```python
from build123d import *

# Parameters (mm, degrees)
F0_R     = 11.1
F0_R_2   = 10.983308
F1_DEPTH = 7
F2_R     = 45.72
F2_R_2   = 41.91
F3_DEPTH = 7


with BuildPart() as f1:
    # F0 (on Top) → F1 (new body)
    with BuildSketch(Plane.XY):
        with BuildLine():
            ThreePointArc((12.948403, 3.187646), (11.548449, 6.6675), (9.234784, 9.619823))
            Line((9.234784, 9.619823), (19.675505, 38.305468))
            ThreePointArc((19.675505, 38.305468), (0, 43.586091), (-19.675505, 38.305468))
            Line((-19.675505, 38.305468), (-9.234784, 9.619823))
            ThreePointArc((-9.234784, 9.619823), (-11.548449, 6.6675), (-12.948403, 3.187646))
            Line((-12.948403, 3.187646), (-43.011261, -2.113247))
            ThreePointArc((-43.011261, -2.113247), (-37.746662, -21.793046), (-23.335756, -36.192221))
            Line((-23.335756, -36.192221), (-3.713619, -12.807469))
            ThreePointArc((-3.713619, -12.807469), (0, -13.335), (3.713619, -12.807469))
            Line((3.713619, -12.807469), (23.335756, -36.192221))
            ThreePointArc((23.335756, -36.192221), (37.746662, -21.793046), (43.011261, -2.113247))
            Line((43.011261, -2.113247), (12.948403, 3.187646))
        make_face()
        with Locations((-22.404077, -12.935)):
            Circle(F0_R, mode=Mode.SUBTRACT)
        with BuildLine():
            ThreePointArc((8.382, 7.276818), (10.398322, 3.883928), (11.1, 0))
            ThreePointArc((11.1, 0), (-10.398322, -3.883928), (8.382, 7.276818))
        make_face(mode=Mode.SUBTRACT)
        with Locations((22.404077, -12.935)):
            Circle(F0_R_2, mode=Mode.SUBTRACT)
        with Locations((0, 25.87)):
            Circle(F0_R, mode=Mode.SUBTRACT)
    extrude(amount=F1_DEPTH)

    # F2 (on Top) → F3 (join)
    with BuildSketch(Plane.XY):
        Circle(F2_R)
        Circle(F2_R_2, mode=Mode.SUBTRACT)
    extrude(amount=F3_DEPTH)


solid = f1.part
```
Can you work these out from the model? Positions are in its coordinate system, mm. A direction names the side the tool comes from. Coordinates: 2 decimals unless noted, no trailing zeros. Write each loop counter-clockwise with the first axis right and the second up, starting at its lowest first coordinate (ties: lowest second). Pieces come first, ordered by that corner, then holes. Notation, with made-up numbers: M 8.25,31.25 L 14.25,31.25 A19 ccw 14.25,45.25 Z; hole C 6,69.25 d10. An arc over 180 degrees is marked long. Answer as CSV lines item,"result".
Item 1: I'm going to push flat-ended pins straight in: P1, Ø4, axis at x = -18.5, z = 2.5, coming from the -Y side; P2, Ø3, axis at x = 9, z = 2.5, coming from the +Y side; P3, Ø13.5, axis at x = 0, y = 0, coming from the +Z side; P4, Ø1.5, axis at x = 12, z = 5, coming from the +Y side. Where does each tip first touch, or does it pass through?
Geometry results:
P1,"stops at y = -42.64"
P2,"stops at y = 45.1"
P3,"passes through"
P4,"stops at y = 44.31"
Item 2: On a 3-axis mill with a long thin cutter (end or side, diameter ignored), from which of +Z, -Z, +X, -X, +Y, -Y can I reach the whole of each face in a straight line? I mean faces 4 (the flat face through (7, -10, 0)), 5 (the flat face through (13.02, -23.9, 3.45)). Say none if no direction works.
Geometry results:
face 4,"-Z, +X, -X, +Y, -Y"
face 5,"+Z, -Z"
Item 3: Imagine slicing it at B-B on y = 29. List the corners of the cut face in (x, z) for me, plus the area to 3 significant figures.
Geometry results:
outline,"M -35.35,0 L -30.26,0 L -30.26,7 L -35.35,7 Z; M -16.29,0 L -10.65,0 L -10.65,7 L -16.29,7 Z; M 10.65,0 L 16.29,0 L 16.29,7 L 10.65,7 Z; M 30.26,0 L 35.35,0 L 35.35,7 L 30.26,7 Z"
area,"150 mm2"
Item 4: We'd pull the mould along X, two halves only. Please class faces 1 (the flat face through (7, -10, 7)), 2 (the flat face through (-14.327, 23.61, 3.451)), 3 (the cylindrical face through (43.61, 13.73, 3.45)): +X half, -X half, draft (parallel to the pull), parting line (faces both ways), or undercut.
Geometry results:
face 1,"draft"
face 2,"undercut"
face 3,"parting line"
Item 5: Imagine slicing it at A-A on x = 0. List the corners of the cut face in (y, z) for me (3 decimals), plus the area to 3 significant figures.
Geometry results:
outline,"M -45.72,0 L -41.91,0 L -41.91,7 L -45.72,7 Z; M -13.335,0 L -11.1,0 L -11.1,7 L -13.335,7 Z; M 11.1,0 L 14.77,0 L 14.77,7 L 11.1,7 Z; M 36.97,0 L 45.72,0 L 45.72,7 L 36.97,7 Z"
area,"129 mm2"
Item 6: Imagine slicing it at D-D on z = 3. List the corners of the cut face in (x, y) for me (1 decimal), plus the area to 3 significant figures.
Geometry results:
outline,"C 0,0 d91.4; hole M -41.9,-1.9 L -12.9,3.2 A13.3 cw -9.2,9.6 L -19.3,37.2 A41.9 ccw Z; hole C -22.4,-12.9 d22.2; hole M -22.6,-35.3 A41.9 ccw 22.6,-35.3 L 3.7,-12.8 A13.3 cw -3.7,-12.8 Z; hole C 0,25.9 d22.2; hole M 8.4,7.3 A11.1 ccw long 11.1,0 A11.1 ccw Z; hole M 9.2,9.6 A13.3 cw 12.9,3.2 L 41.9,-1.9 A41.9 ccw 19.3,37.2 Z; hole C 22.4,-12.9 d22"
area,"2,650 mm2"
Item 7: Please list where these lines run through material, in increasing order: line 1 along Y through (x, z) = (28.5, 5.25); line 2 along X through (y, z) = (6.5, 5.5); line 3 along Y through (x, z) = (9, 5.75).
Geometry results:
line 1,"y = -35.75 to -22.07, -3.8 to 0.45, 30.73 to 35.75"
line 2,"x = -45.26 to -41.4, -11.64 to -9, 9 to 11.64, 41.4 to 45.26"
line 3,"y = -44.83 to -40.93, -19.11 to -6.5, 6.5 to 19.37, 32.37 to 44.83"
Item 8: Imagine slicing it at C-C on x = 38. List the corners of the cut face in (y, z) for me, plus the area to 3 significant figures.
Geometry results:
outline,"M -25.42,0 L -1.23,0 L -1.23,7 L -25.42,7 Z; M 17.68,0 L 25.42,0 L 25.42,7 L 17.68,7 Z"
area,"224 mm2"
